Part model, mm, in its own coordinate system. Face numbers are marked on the shaded views. Coordinates: 2 decimals unless noted, no trailing zeros. Loops run counter-clockwise (first coordinate to the right, second up) from the corner with the lowest first, then second, coordinate; pieces in that order, holes last. Notation, with made-up numbers: M 80.25,-21.5 L 109.25,-21.5 A19 ccw 109.25,4.5 Z; hole C 13.5,53.25 d7. An arc over 180 degrees is marked long. Answer as a JSON object with one key per item and string values. Group by question number.
1. Saw through at B-B on y = 31.75. Count the separate pieces of the cut face and the enclosed holes in it, then the cut area to 3 significant figures.
2. Mould opens along Y. For the marked faces 1, 2 and 3 say: released by +Y, released by -Y, zero draft, split by the parting line, or undercut.
3. Drill centre lines: L1, parallel to X at y = 31.75, z = -13.5; L2, parallel to Z at x = 0, y = -23.5; L3, parallel to Y at x = -36.5, z = -9. Where is each one in solid material? Low to high.
4. Saw through at C-C on x = 31.75. Write the cut outline in (y, z), then the cut area to 3 significant figures.
5. Drop flat-ended pins along their axis: pin 1 Ø20.5 at (x, z) = (0, 0) entering from +Y; pin 2 Ø10 at (x, y) = (-0.5, -10) entering from +Z; pin 3 Ø15.5 at (x, y) = (31.75, 31.75) entering from +Z; pin 4 Ø17.5 at (x, y) = (-31.75, 31.75) entering from +Z. Give the stop position or say it passes through.
6. Saw through at D-D on y = -11. Write the cut outline in (x, z), then the cut area to 3 significant figures.
7. Saw through at A-A on z = 0. Write the cut outline in (x, y).
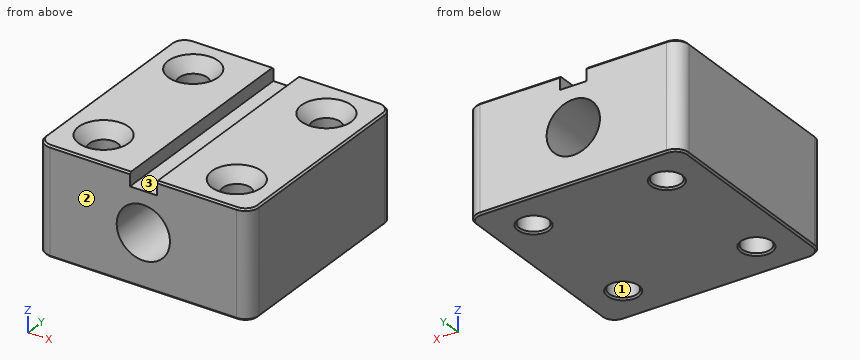
from build123d import *

# Parameters (mm, degrees)
F1_DEPTH       = 50.8
F3_D           = 13.49248
F3_CSINK_D     = 23.8252
F3_CSINK_ANGLE = 82
F4_R           = 6.35
F5_SIZE        = 0.8128
F7_D           = 25.4


with BuildPart() as f1:
    # F0 (on Front) → F1 (new body, symmetric)
    with BuildSketch(Plane.XZ):
        Polygon((-6.35, 25.4), (-50.8, 25.4), (-50.8, -25.4), (50.8, -25.4), (50.8, 25.4), (6.4515996888, 25.4), (6.4515996888, 19.05), (-6.35, 19.05), align=None)
    extrude(amount=F1_DEPTH, both=True)

    # F3 (through all)
    with Locations(Plane.XY.offset(25.4)):
        with Locations((-31.75, 31.75), (31.75, 31.75), (-31.75, -31.75), (31.75, -31.75)):
            CounterSinkHole(F3_D / 2, F3_CSINK_D / 2, counter_sink_angle=F3_CSINK_ANGLE)

    # F4
    f4_edges = [f1.edges().sort_by_distance(p)[0] for p in [
        (50.8, 50.8, 0),
        (50.8, -50.8, 0),
        (-50.8, -50.8, 0),
        (-50.8, 50.8, 0),
    ]]
    fillet(f4_edges, radius=F4_R)

    # F5
    f5_edges = [f1.edges().sort_by_distance(p)[0] for p in [
        (-50.8, 0, 25.4),
        (50.8, 0, 25.4),
        (-25.4, 50.8, 25.4),
        (25.4508, 50.8, 25.4),
        (-25.4, -50.8, 25.4),
        (25.4508, -50.8, 25.4),
        (-50.8, 0, -25.4),
        (-48.940128, 48.940128, -25.4),
        (-48.940128, -48.940128, -25.4),
        (0, 50.8, -25.4),
        (0, -50.8, -25.4),
        (48.940128, 48.940128, -25.4),
        (48.940128, -48.940128, -25.4),
        (50.8, 0, -25.4),
        (-38.49624, 31.75, -25.4),
        (25.00376, 31.75, -25.4),
        (-38.49624, -31.75, -25.4),
        (25.00376, -31.75, -25.4),
    ]]
    chamfer(f5_edges, length=F5_SIZE)

    # F7 (through all)
    with Locations(Plane.XZ.offset(50.8)):
        with Locations((0, 0)):
            Hole(F7_D / 2)


solid = f1.part
Outcome:
{
 "1": {"separate pieces": "3", "enclosed holes": "1", "area": "3,140 mm²"},
 "2": {"face 1": "undercut", "face 2": "released by -Y", "face 3": "zero draft"},
 "3": {"L1": "x = -50.8 to -38.5, -25 to 25, 38.5 to 50.8", "L2": "z = -25.4 to -12.7, 12.7 to 19.05", "L3": "y = -50.8 to -36.54, -26.96 to 26.96, 36.54 to 50.8"},
 "4": {"outline": "M -50.8,-24.59 L -49.99,-25.4 L -39.31,-25.4 L -38.5,-24.59 L -38.5,19.46 L -43.66,25.4 L -49.99,25.4 L -50.8,24.59 Z; M -25,-24.59 L -24.19,-25.4 L 24.19,-25.4 L 25,-24.59 L 25,19.46 L 19.84,25.4 L -19.84,25.4 L -25,19.46 Z; M 38.5,-24.59 L 39.31,-25.4 L 49.99,-25.4 L 50.8,-24.59 L 50.8,24.59 L 49.99,25.4 L 43.66,25.4 L 38.5,19.46 Z", "area": "3,730 mm²"},
 "5": {"pin 1": "passes through", "pin 2": "stops at z = 19.05", "pin 3": "stops at z = 20.61", "pin 4": "stops at z = 21.76"},
 "6": {"outline": "M -50.8,-24.59 L -49.99,-25.4 L 49.99,-25.4 L 50.8,-24.59 L 50.8,24.59 L 49.99,25.4 L 6.45,25.4 L 6.45,19.05 L -6.35,19.05 L -6.35,25.4 L -49.99,25.4 L -50.8,24.59 Z; hole C 0,0 d25.4", "area": "4,570 mm²"},
 "7": {"outline": "M -50.8,-44.45 A6.35 ccw -44.45,-50.8 L -12.7,-50.8 L -12.7,50.8 L -44.45,50.8 A6.35 ccw -50.8,44.45 Z; M 12.7,-50.8 L 44.45,-50.8 A6.35 ccw 50.8,-44.45 L 50.8,44.45 A6.35 ccw 44.45,50.8 L 12.7,50.8 Z; hole C -31.75,-31.75 d13.49; hole C -31.75,31.75 d13.49; hole C 31.75,-31.75 d13.49; hole C 31.75,31.75 d13.49"}
}
